Could you check a few things on this drawing? It's one solid part, dimensions in mm from its lowest x, y, z. Coordinates: 2 decimals unless noted, no trailing zeros. Write each loop counter-clockwise with the first axis right and the second up, starting at its lowest first coordinate (ties: lowest second). Pieces come first, ordered by that corner, then holes.
Item 1: I want a section at B-B (x = 44). Please give me the cut outline in (y, z), and give its area (3 significant figures).
Item 2: I'm going to push flat-ended pins straight in: P1, Ø1, axis at y = 4, z = 69.5, coming from the +X side; P2, Ø1.5, axis at x = 41, y = 2, coming from the +Z side. Where does each tip first touch, or does it pass through?
Item 3: I want a section at C-C (z = 20). Please give me the cut outline in (x, y) (3 decimals), and give its area (3 significant figures).
Item 4: I want a section at A-A (y = 2.5). Please give me the cut outline in (x, z) (3 decimals).
Item 5: I want a section at D-D (z = 79). Please give me the cut outline in (x, y), and give its area (3 significant figures).
Item 6: Please list where these lines run through material, in increasing order: line 1 (Z direction, x = 47, y = 3); line 2 (Z direction, x = 54, y = 1.5); line 3 (Z direction, x = 57, y = 0.5).
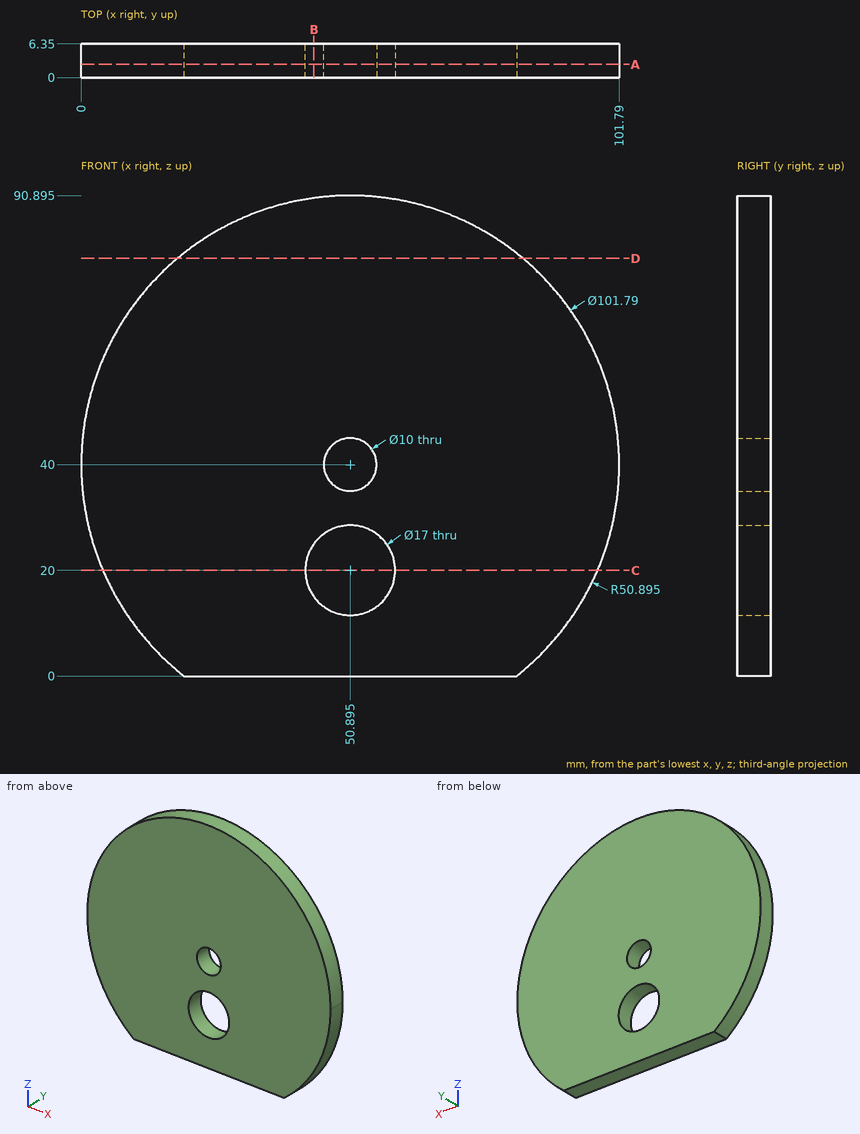
Answer:
1. outline: (0, 0) - (6.35, 0) - (6.35, 15.03) - (0, 15.03) - close; (0, 24.97) - (6.35, 24.97) - (6.35, 90.43) - (0, 90.43) - close
1. area: 511 mm2
2. P1: stops at x = 92.72
2. P2: stops at z = 90.07
3. outline: (4.094, 0) - (42.395, 0) - (42.395, 6.35) - (4.094, 6.35) - close; (59.395, 0) - (97.696, 0) - (97.696, 6.35) - (59.395, 6.35) - close
3. area: 486 mm2
4. outline: (19.426, 0) - (82.364, 0) arc R50.895 ccw (long way) to start; hole circle Ø17 at (50.895, 20); hole circle Ø10 at (50.895, 40)
5. outline: (18.19, 0) - (83.6, 0) - (83.6, 6.35) - (18.19, 6.35) - close
5. area: 415 mm2
6. line 1: z = 0 to 12.44, 27.56 to 36.86, 43.14 to 90.75
6. line 2: z = 0 to 12.09, 27.91 to 36.08, 43.92 to 90.8
6. line 3: z = 0 to 14.09, 25.91 to 90.53
